Input: dimensioned drawing with shaded views. Units: mm. Origin: part minimum x, y, z. A direction names the side the tool comes from. Give positions to 0.01 mm unless a question says otherwise; leave off trailing zeros. Order: outer loops, then holes, each group sorted by start corner. A loop starts at its lowest first (then second) coordinate and runs counter-clockwise, first axis right, second up. Notation, with made-up numbers: (-4.5, 33) - (47.5, 33) arc R26 cw to (47.5, 50) - close; hole circle Ø4 at (-15.5, 20.25). An arc over 180 degrees is marked (long way). Use a Markdown table: item, result.
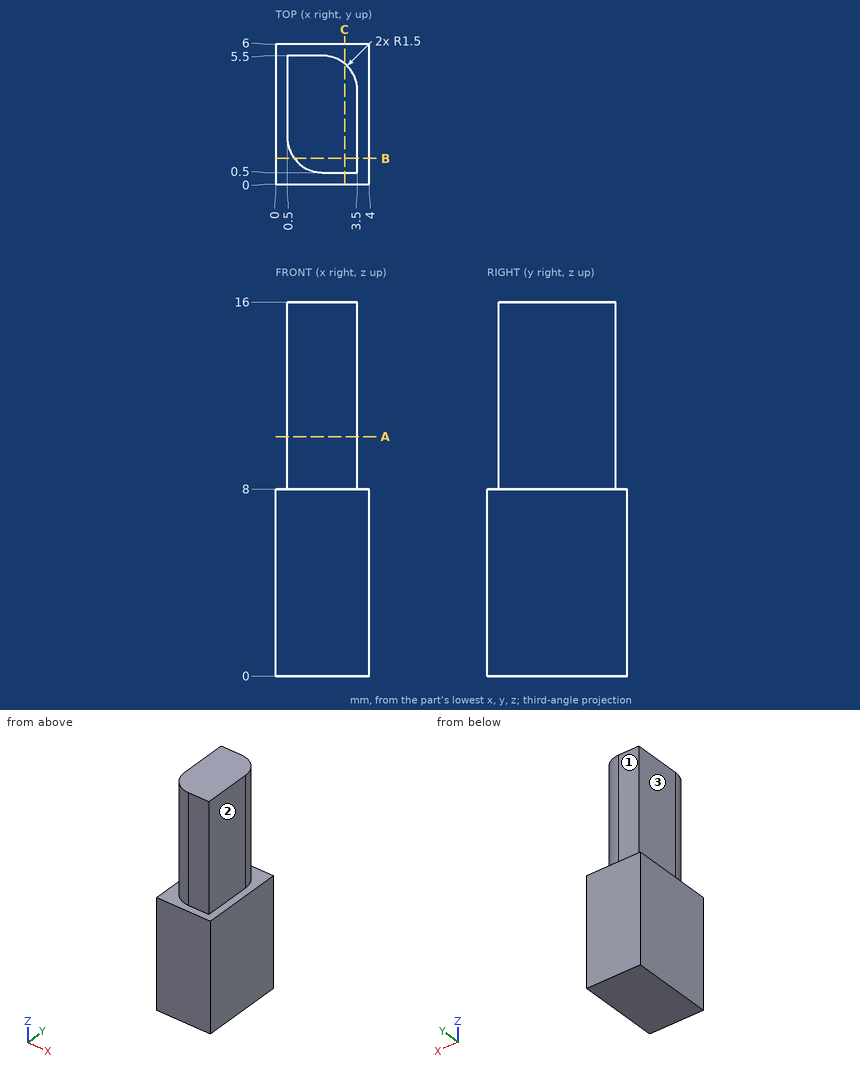
1. Set-up query: the marked faces 1, 2 and 3. Return all of +Z, -Z, +X, -X, +Y, -Y with unobstructed straight access to the full face (end or side cutting, diameter ignored); none if empty.
Response:
| item | result |
|---|---|
| face 1 | +Z, +X, -X, +Y |
| face 2 | +Z, +X, +Y, -Y |
| face 3 | +Z, -X, +Y, -Y |
2. Section query C-C (x = 2.95). Return loops of the section in (y, z), then the cut area to 3 significant figures.
Response:
| item | result |
|---|---|
| outline | (0, 0) - (6, 0) - (6, 8) - (5.16, 8) - (5.16, 16) - (0.5, 16) - (0.5, 8) - (0, 8) - close |
| area | 85.3 mm^2 |
3. Section query A-A (z = 10.25). Return loops of the section in (x, y).
Response:
| item | result |
|---|---|
| outline | (0.5, 2) arc R1.5 ccw to (2, 0.5) - (3.5, 0.5) - (3.5, 4) arc R1.5 ccw to (2, 5.5) - (0.5, 5.5) - close |
4. Pin query (flat end, axial travel): pin 1 (1.2 mm diameter, centred on x = 2.5, z = 13.5, fed in from -Y); pin 2 (3 mm diameter, centred on y = 5, z = 13.5, fed in from +X); pin 3 (2 mm diameter, centred on x = 0.5, z = 8.5, fed in from +Y); pin 4 (1.8 mm diameter, centred on y = 4.5, z = 12.5, fed in from -X). Return the tip coordinate at first contact, or that it passes through.
Response:
| item | result |
|---|---|
| pin 1 | stops at y = 0.5 |
| pin 2 | stops at x = 3.5 |
| pin 3 | stops at y = 6 |
| pin 4 | stops at x = 0.5 |
5. Material intervals for line 1 along Z through (x, y) = (0.3, 1.8); line 2 along Y through (x, z) = (2, 9); line 3 along X through (y, z) = (3.5, 12.5), sorted ascending.
Response:
| item | result |
|---|---|
| line 1 | z = 0 to 8 |
| line 2 | y = 0.5 to 5.5 |
| line 3 | x = 0.5 to 3.5 |
6. Section query B-B (y = 1.1). Return loops of the section in (x, z), then the cut area to 3 significant figures.
Response:
| item | result |
|---|---|
| outline | (0, 0) - (4, 0) - (4, 8) - (3.5, 8) - (3.5, 16) - (0.8, 16) - (0.8, 8) - (0, 8) - close |
| area | 53.6 mm^2 |
